```python
from build123d import *

# Parameters (mm, degrees)
SKETCH_2_RX            = 3
SKETCH_2_RY            = 2
EXTRUDE_1_DEPTH        = 50
SKETCH_5_W             = 1.5
SKETCH_5_H             = 1
CUT_EXTRUDE_2_DEPTH    = 25
CUT_EXTRUDE_4_DEPTH    = 25
PATTERN_START          = 97.264960027
PATTERN_LINEAR_1_DEPTH = 0.850363271
PATTERN_LINEAR_2_DEPTH = 0.850363271


# Read off the part's stored shape, not the designer's step: 阵列(线性)1, 阵列(线性)2
with BuildPart() as part:
    # 草图2 → 凸台-拉伸1 (new body)
    with BuildSketch(Plane(origin=(0, 0, 0), x_dir=(0, 0, -1), z_dir=(1, 0, 0))):
        with Locations(Location((-5.2411758, 96.567762113), (0, 0, 8.868937921))):
            Ellipse(SKETCH_2_RX, SKETCH_2_RY)
    extrude(amount=EXTRUDE_1_DEPTH)

    # 草图5 → 切除-拉伸2 (cut, symmetric)
    with BuildSketch(Plane(origin=(0, 1.757367098, -10.542320534), x_dir=(1, 0, 0), z_dir=(0, -0.1644275429715825, 0.986389164129619))):
        with Locations((5.25, 97.615322624)):
            Rectangle(SKETCH_5_W, SKETCH_5_H)
    cut_extrude_2 = extrude(amount=CUT_EXTRUDE_2_DEPTH, both=True, mode=Mode.SUBTRACT)

    # 镜向2: 切除-拉伸2 across plane
    add(cut_extrude_2.mirror(Plane(origin=(25, 0, 0), x_dir=(0, 0, 1), z_dir=(1, 0, 0))), mode=Mode.SUBTRACT)

    # 草图7 → 切除-拉伸4 (cut, symmetric)
    with BuildSketch(Plane(origin=(23.377948952, 2.219322141, -13.31355606), x_dir=(0.49999999999999795, -0.14239842929524804, 0.8542380741539494), z_dir=(-0.8660254037844399, -0.0822137714857909, 0.4931945820648075))):
        Polygon((3.244102096, 98.345137773), (4.244102028, 98.34550487), (4.244102028, 97.264960027), (3.244102096, 97.264960027), align=None)
    extrude(amount=CUT_EXTRUDE_4_DEPTH, both=True, mode=Mode.SUBTRACT)

    # 阵列(线性)1 outline → 阵列(线性)1 (cut)
    with BuildSketch(Plane(origin=(0, 0, 0), x_dir=(1, 0, 0), z_dir=(0, 0.986389164129618, 0.164427542971589)).offset(PATTERN_START)):
        Polygon((32.758607465, 8.239021249), (41.261648564, 13.148254316), (43, 14.151891985), (43, 15), (42.468966305, 15), (39.261648698, 13.148254316), (30.7586076, 8.239021249), (29, 7.223688678), (29, 7), (30.61255971, 7), align=None)
    extrude(amount=PATTERN_LINEAR_1_DEPTH, mode=Mode.SUBTRACT)

    # 阵列(线性)2 outline → 阵列(线性)2 (cut)
    with BuildSketch(Plane(origin=(0, 0, 0), x_dir=(1, 0, 0), z_dir=(0, 0.986389164129618, 0.164427542971589)).offset(PATTERN_START)):
        Polygon((12.758607465, 8.239021249), (21.261648564, 13.148254316), (23, 14.151891985), (23, 15), (22.468966305, 15), (19.261648698, 13.148254316), (10.7586076, 8.239021249), (9, 7.223688678), (9, 7), (10.61255971, 7), align=None)
    extrude(amount=PATTERN_LINEAR_2_DEPTH, mode=Mode.SUBTRACT)


solid = part.part
```
Part model, mm, in its own coordinate system. A direction names the side the tool comes from. Round coordinates to 2 decimals unless told otherwise and drop trailing zeros.
1. Two-plate mould, pull along Y, no slides. Class faces 5 (the face through (44.76, 97.546, 5.454)), 6 (the face through (6, 98, 6)), 7 (the face through (15.07, 98.026, 5.465)): pulls with the +Y half, pulls with the -Y half, needs draft (parallel to the pull), parting line crosses it, or undercut.
Solutions:
face 5: pulls with the +Y half
face 6: needs draft
face 7: undercut
2. Flat gauge pin, fed straight in: pin 1 (1.5 mm diameter, centred on x = 15.5, z = 4.5, fed in from -Y). Where does the tip first touch, or does it go through?
Solutions:
pin 1: stops at y = 94.55
3. 3-axis set-ups, long thin cutter, end or side, ignore diameter. For faces 1 (the face through (27, 98, 5.5)), 2 (the face through (50, 97, 5)), 3 (the face through (45.5, 98, 6)), 4 (the face through (25, 98, 5.5)): which of +Z, -Z, +X, -X, +Y, -Y reach the whole face in a straight line?
Solutions:
face 1: +Y
face 2: +Z, -Z, +X, +Y, -Y
face 3: +Z, +Y
face 4: none
4. Drill centre lines: line 1 along X through (y, z) = (97.75, 7.1); line 2 along X through (y, z) = (98.2, 3.9); line 3 along Y through (x, z) = (39, 3.05). Where is each one in solid material? Low to high.
Solutions:
line 1: x = 0 to 4.5, 6 to 12.2, 14.2 to 22.2, 24.2 to 32.2, 34.2 to 44, 45.5 to 50
line 2: x = 0 to 4.5, 6 to 17.79, 19.79 to 27.79, 29.79 to 37.79, 39.79 to 44, 45.5 to 50
line 3: y = 95.39 to 98.12
